from build123d import *

# Parameters (mm, degrees)
ESBO_O1_W               = 400
ESBO_O1_H               = 300
FLANGE_BASE1_DEPTH      = 2
DOBRA_START             = -200
DOBRA_ESBO_ADA1_DEPTH   = 400
DOBRA_ESBO_ADA1_2_DEPTH = 400
ESBO_O9_W               = 25
ESBO_O9_H               = 25
ESBO_O9_W_2             = 50
CORTE_EXTRUS_O1_DEPTH   = 2


# Read off the part's stored shape, not the designer's step: Dobra esboçada1
# Sheet-metal steps are written as plain solids
with BuildPart() as part:
    # Esboço1 → Flange-base1 (new body)
    with BuildSketch(Plane(origin=(0, 0, 0), x_dir=(1, 0, 0), z_dir=(0, 1, 0))):
        with Locations((0, 150)):
            Rectangle(ESBO_O1_W, ESBO_O1_H)
    extrude(amount=-FLANGE_BASE1_DEPTH)

    # Dobra esboçada1 outline → Dobra esboçada1 (cut)
    with BuildSketch(Plane.YZ.offset(DOBRA_START)):
        with BuildLine():
            Line((-1.198468417, -48.746892808), (0, -47.548424391))
            Line((0, -47.548424391), (0, 0))
            Line((0, 0), (-2, 0))
            Line((-2, 0), (-2, -50.681961225))
            ThreePointArc((-2, -50.681961225), (-1.791688729, -49.634709744), (-1.198468417, -48.746892808))
        make_face()
    extrude(amount=DOBRA_ESBO_ADA1_DEPTH, mode=Mode.SUBTRACT)

    # Dobra esbo_ada1 2 outline → Dobra esbo_ada1 2 (add)
    with BuildSketch(Plane.YZ.offset(DOBRA_START)):
        with BuildLine():
            Line((35.088864797, -15.287986718), (33.674651235, -13.873773155))
            Line((33.674651235, -13.873773155), (0, -47.548424391))
            Line((0, -47.548424391), (0, -50.681961225))
            ThreePointArc((0, -50.681961225), (0.056070336, -50.400076609), (0.215745145, -50.16110637))
            Line((0.215745145, -50.16110637), (35.088864797, -15.287986718))
        make_face()
    extrude(amount=DOBRA_ESBO_ADA1_2_DEPTH)

    # Esboço9 → Corte-extrusão1 (cut)
    with BuildSketch(Plane(origin=(0, 25.188425758, -25.188425758), x_dir=(1, 0, 0), z_dir=(0, 0.7071067811865464, -0.7071067811865488))):
        with Locations((-187.5, -1.501335164)):
            Rectangle(ESBO_O9_W, ESBO_O9_H)
        with Locations((0, -1.501335164)):
            Rectangle(ESBO_O9_W_2, ESBO_O9_H)
        with Locations((187.5, -1.501335164)):
            Rectangle(ESBO_O9_W, ESBO_O9_H)
    extrude(amount=-CORTE_EXTRUS_O1_DEPTH, mode=Mode.SUBTRACT)


solid = part.part
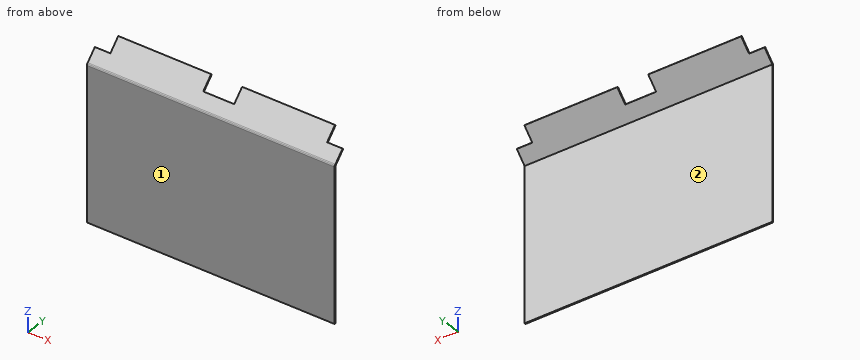
Geometry check sheet. Reference: the model listing, model coordinates, mm. Face numbers are marked on the shaded views. A direction names the side the tool comes from. Give positions to 0.01 mm unless a question says otherwise; leave off trailing zeros. Write each loop counter-clockwise with the first axis right and the second up, starting at its lowest first coordinate (ties: lowest second). Pieces come first, ordered by that corner, then holes. Notation, with made-up numbers: M 51,-10 L 65,-10 A9 ccw 65,0 Z; hole C 15,6 d10. An arc over 180 degrees is marked long. One line per question, with ' | ' between items.
1. Scan lines: line 1 along Y through (x, z) = (-66, -83); line 2 along Y through (x, z) = (-135.5, -41); line 3 along Z through (x, y) = (-7, 1). Record each from-to range of solid material in increasing order. Write a range as from..to.
Ans:
line 1: -2..0 | line 2: 6.55..9.38 | line 3: -49.38..-46.55
2. Gauge pin test, flat ends, axial feed: pin 1 (8 mm diameter, centred on x = 39.5, z = -125, fed in from +Y); pin 2 (3 mm diameter, centred on x = 109, y = 15.5, fed in from -Z); pin 3 (9.5 mm diameter, centred on y = 27, z = -27, fed in from +X). Record the tip position at first contact, or that the pin passes through.
Ans:
pin 1: y = 0 | pin 2: z = -36.38 | pin 3: x = 175
3. Set-up check for the marked faces 1 and 2: record each of +Z, -Z, +X, -X, +Y, -Y from which the full face is reachable in a straight line by a thin tool's end or side.
Ans:
face 1: +Z, -Z, +X, -X, -Y | face 2: -Z, +X, -X, +Y
4. Cross-section at C-C (z = -243). Enter the section's corners in (x, y), plus the area to 3 significant figures.
Ans:
outline: M -200,-2 L 200,-2 L 200,0 L -200,0 Z | area: 800 mm2
5. Cross-section at B-B (x = 167.5). Enter the section's corners in (y, z), plus the area to 3 significant figures.
Ans:
outline: M -2,-300 L 0,-300 L 0,-50.68 A0.74 cw 0.22,-50.16 L 35.09,-15.29 L 33.67,-13.87 L -1.2,-48.75 A2.74 ccw -2,-50.68 Z | area: 600 mm2
6. Cross-section at A-A (y = 26). Enter the section's corners in (x, z).
Ans:
outline: M -175,-24.38 L -25,-24.38 L -25,-21.55 L -175,-21.55 Z; M 25,-24.38 L 175,-24.38 L 175,-21.55 L 25,-21.55 Z
